CAD build for the part. Positions are in the model's coordinates, mm. Face numbers are marked on the shaded views. Coordinates: 2 decimals unless noted, no trailing zeros. Order: outer loops, then holes, each group sorted by start corner. A loop starts at its lowest first (then second) coordinate and runs counter-clockwise, first axis right, second up. Notation, with made-up numbers: (59, 36.5) -> (111, 36.5) arc R13 cw to (111, 49.5) -> close; hole circle Ø10 at (79.25, 6). An arc over 180 degrees is marked (long way). Use one line per item in the form item = value. Start each with the question number.
from build123d import *

# Parameters (mm, degrees)
EXTRUDE_1_DEPTH     = 1.5
FILLET_1_R          = 2
SKETCH_2_W          = 12
SKETCH_2_H          = 3.5
CUT_EXTRUDE_1_DEPTH = 1.5
SKETCH_3_W          = 2.5
SKETCH_3_H          = 2
EXTRUDE_2_DEPTH     = 2.3
EXTRUDE_2_TAPER     = 1
HOLE_WIZARD_M2_1_D  = 2.2
FILLET_2_R          = 1.5


with BuildPart() as part:
    # 草图1 → 凸台-拉伸1 (new body)
    with BuildSketch(Plane.XY):
        with BuildLine():
            Line((-25, -3.5), (25, -3.5))
            ThreePointArc((25, -3.5), (26.854367709, -2.249213187), (26.389316741, -0.061320399))
            Line((26.389316741, -0.061320399), (23.06389712, 3.15))
            Line((23.06389712, 3.15), (-23.06389712, 3.15))
            Line((-23.06389712, 3.15), (-26.389316741, -0.061320399))
            ThreePointArc((-26.389316741, -0.061320399), (-26.854367709, -2.249213187), (-25, -3.5))
        make_face()
    extrude(amount=-EXTRUDE_1_DEPTH)

    # 圆角1
    fillet_1_edges = [part.edges().sort_by_distance(p)[0] for p in [
        (-23.06389712, 3.15, -0.75),
        (23.06389712, 3.15, -0.75),
    ]]
    fillet(fillet_1_edges, radius=FILLET_1_R)

    # 草图2 → 切除-拉伸1 (cut)
    with BuildSketch(Plane.XY):
        with Locations((-4, -1.75)):
            Rectangle(SKETCH_2_W, SKETCH_2_H)
    extrude(amount=-CUT_EXTRUDE_1_DEPTH, mode=Mode.SUBTRACT)

    # 草图3 → 凸台-拉伸2 (add)
    with BuildSketch(Plane(origin=(0, 0, -1.5), x_dir=(-1, 0, 0), z_dir=(0, 0, -1))):
        with Locations((16.9, 2.1)):
            Rectangle(SKETCH_3_W, SKETCH_3_H)
    extrude_2 = extrude(amount=EXTRUDE_2_DEPTH, taper=EXTRUDE_2_TAPER)

    # M2 间隙孔1 (through all)
    with Locations(Plane(origin=(0, 0, -1.5), x_dir=(-1, 0, 0), z_dir=(0, 0, -1))):
        with Locations((25, -1.5)):
            hole_wizard_m2_1 = Hole(HOLE_WIZARD_M2_1_D / 2)

    # 镜向1: 凸台-拉伸2, M2 间隙孔1 across plane
    add(extrude_2.mirror(Plane(origin=(0, 0, 0), x_dir=(0, 0, 1), z_dir=(1, 0, 0))))
    add(hole_wizard_m2_1.mirror(Plane(origin=(0, 0, 0), x_dir=(0, 0, 1), z_dir=(1, 0, 0))), mode=Mode.SUBTRACT)

    # 圆角2
    fillet_2_edges = [part.edges().sort_by_distance(p)[0] for p in [
        (2, 0, -0.75),
        (2, -3.5, -0.75),
        (-10, -3.5, -0.75),
        (-10, 0, -0.75),
    ]]
    fillet(fillet_2_edges, radius=FILLET_2_R)


solid = part.part
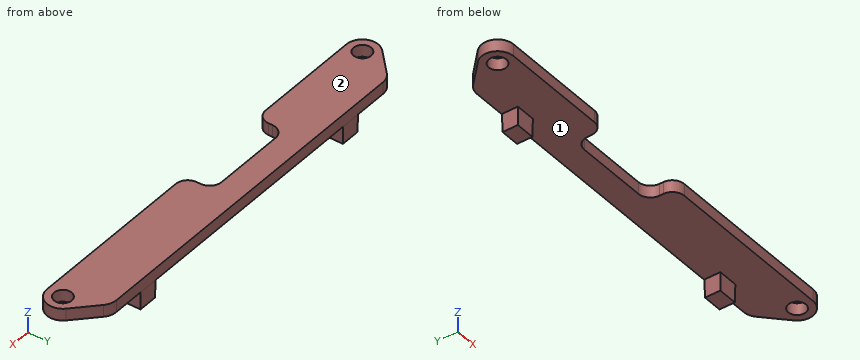
1) Probe L1, parallel to Z at x = 12.5, y = 1; L2, parallel to Y at x = -3, z = -0.95; L3, parallel to Y at x = -24, z = -0.85. List the from-to ranges inside material, lowest first.
2) Cut at A-A on z = -0.7. Give the cut face in (x, y), then the cut area to 3 significant figures.
3) Cut at B-B on y = -1. Give the cut face in (x, z), then the cut area to 3 significant figures.
4) Drop flat-ended pins along their axis: P1, Ø2.5, axis at x = 25, y = -1.5, coming from the -Z side; P2, Ø0.6, axis at y = -2, z = -1, coming from the +X side. Give the stop position or say it passes through.
5) Cut at C-C on x = 12.5. Give the cut face in (y, z), then the cut area to 4 significant figures.
6) Cut at D-D on x = -10.5. Give the cut face in (y, z).
7) Two-plate mould, pull along X, no slides. Class the marked faces 1 and 2: released by +X, released by -X, zero draft, split by the parting line, or undercut.
Values follow:
q1.L1 = -1.5 to 0
q1.L2 = 0 to 3.15
q1.L3 = -3.5 to -1.96, -1.04 to 2.25
q2.outline = (-26.39, -0.06) arc R2 ccw to (-25, -3.5) -> (-11.5, -3.5) arc R1.5 ccw to (-10, -2) -> (-10, -1.5) arc R1.5 cw to (-8.5, 0) -> (0.5, 0) arc R1.5 cw to (2, -1.5) -> (2, -2) arc R1.5 ccw to (3.5, -3.5) -> (25, -3.5) arc R2 ccw to (26.39, -0.06) -> (23.65, 2.59) arc R2 ccw to (22.26, 3.15) -> (-22.26, 3.15) arc R2 ccw to (-23.65, 2.59) -> close; hole circle Ø2.2 at (-25, -1.5); hole circle Ø2.2 at (25, -1.5)
q2.area = 292 mm^2
q3.outline = (-26.94, -1.5) -> (-25.98, -1.5) -> (-25.98, 0) -> (-26.94, 0) -> close; (-24.02, -1.5) -> (-9.91, -1.5) -> (-9.91, 0) -> (-24.02, 0) -> close; (1.91, -1.5) -> (24.02, -1.5) -> (24.02, 0) -> (1.91, 0) -> close; (25.98, -1.5) -> (26.94, -1.5) -> (26.94, 0) -> (25.98, 0) -> close
q3.area = 57.2 mm^2
q4.P1 = -1.5
q4.P2 = 26.99
q5.outline = (-3.5, -1.5) -> (3.15, -1.5) -> (3.15, 0) -> (-3.5, 0) -> close
q5.area = 9.975 mm^2
q6.outline = (-3.12, -1.5) -> (3.15, -1.5) -> (3.15, 0) -> (-3.12, 0) -> close
q7.face_1 = undercut
q7.face_2 = zero draft
